```python
from build123d import *

# Parameters (mm, degrees)
ESQUISSE1_R                                        = 19
BOSS_EXTRU_1_DEPTH                                 = 2.1
ESQUISSE2_R                                        = 10
BOSS_EXTRU_2_DEPTH                                 = 6
ESQUISSE4_R                                        = 4.5
ENL_V_MAT_EXTRU_1_DEPTH                            = 21
ESQUISSE5_R                                        = 6
ENL_V_MAT_EXTRU_2_DEPTH                            = 7.2
ENL_V_MAT_EXTRU_3_DEPTH                            = 4.2
ENL_V_MAT_EXTRU_3_DEPTH_BACK                       = 10
CONG_1_R                                           = 4
ESQUISSE7_R                                        = 1.6
ENL_V_MAT_EXTRU_4_DEPTH                            = 4.2
CONG_2_R                                           = 4
ESQUISSE8_W                                        = 24.922206
ESQUISSE8_H                                        = 11.327448
ENL_V_MAT_EXTRU_5_DEPTH                            = 25
ESQUISSE9_R                                        = 4
ESQUISSE9_R_2                                      = 1.6
BOSS_EXTRU_4_DEPTH                                 = 5
CHAMBRAGE_POUR_VIS_T_TE_RONDE_BOMB_E_M_D           = 3.5
CHAMBRAGE_POUR_VIS_T_TE_RONDE_BOMB_E_M_DEPTH       = 6.948494
CHAMBRAGE_POUR_VIS_T_TE_RONDE_BOMB_E_M_CBORE_D     = 4.35
CHAMBRAGE_POUR_VIS_T_TE_RONDE_BOMB_E_M_CBORE_DEPTH = 4.8
CHAMBRAGE_POUR_VIS_T_TE_RONDE_BOMB_E_M_TIP         = 1.051506


with BuildPart() as part:
    # Esquisse1 → Boss.-Extru.1 (new body)
    with BuildSketch(Plane.XY):
        Circle(ESQUISSE1_R)
    extrude(amount=BOSS_EXTRU_1_DEPTH)

    # Esquisse2 → Boss.-Extru.2 (add)
    with BuildSketch(Plane.XY.offset(2.1)):
        Circle(ESQUISSE2_R)
    extrude(amount=BOSS_EXTRU_2_DEPTH)

    # Esquisse3 → Révolution1 (revolve)
    with BuildSketch(Plane(origin=(0, 0, 0), x_dir=(0, 0, -1), z_dir=(1, 0, 0))):
        Polygon((7.5, 0), (0, -11.25), (0, 0), align=None)
    revolve(axis=Axis((0, 0, 0), (0, 0, -1)))

    # Esquisse4 → Enlèv. mat.-Extru.1 (cut)
    with BuildSketch(Plane(origin=(0, 3.461538, -5.192308), x_dir=(0, 0.83205, 0.5547), z_dir=(0, 0.5547, -0.83205))):
        with Locations((2.600157, 0)):
            Circle(ESQUISSE4_R)
    extrude(amount=-ENL_V_MAT_EXTRU_1_DEPTH, mode=Mode.SUBTRACT)

    # Esquisse5 → Enlèv. mat.-Extru.2 (cut)
    with BuildSketch(Plane(origin=(0, 3.461538, -5.192308), x_dir=(0, 0.83205, 0.5547), z_dir=(0, 0.5547, -0.83205))):
        with Locations((2.600157, 0)):
            Circle(ESQUISSE5_R)
    extrude(amount=-ENL_V_MAT_EXTRU_2_DEPTH, mode=Mode.SUBTRACT)

    # Esquisse6 → Enlèv. mat.-Extru.3 (cut, two sides)
    with BuildSketch(Plane(origin=(0, 0, 0), x_dir=(1, 0, 0), z_dir=(0, 1, 0))) as enl_v_mat_extru_3_sk:
        with BuildLine():
            Line((2.748075, 5.66795), (0, 7.5))
            Line((0, 7.5), (-2.748075, 5.66795))
            ThreePointArc((-2.748075, 5.66795), (0, 6.5), (2.748075, 5.66795))
        make_face()
    extrude(amount=ENL_V_MAT_EXTRU_3_DEPTH, mode=Mode.SUBTRACT)
    extrude(enl_v_mat_extru_3_sk.sketch, amount=-ENL_V_MAT_EXTRU_3_DEPTH_BACK, mode=Mode.SUBTRACT)

    # Congé1
    cong_1_edges = [part.edges().sort_by_distance(p)[0] for p in [
        (-1.569953, -1.039687, -6.244664),
    ]]
    fillet(cong_1_edges, radius=CONG_1_R)

    # Esquisse7 → Enlèv. mat.-Extru.4 (cut)
    with BuildSketch(Plane(origin=(0, 0, 0), x_dir=(-1, 0, 0), z_dir=(0, 0, -1))):
        with Locations((-15, 0)):
            Circle(ESQUISSE7_R)
        with Locations((15, 0)):
            Circle(ESQUISSE7_R)
    extrude(amount=-ENL_V_MAT_EXTRU_4_DEPTH, mode=Mode.SUBTRACT)

    # Congé2
    cong_2_edges = [part.edges().sort_by_distance(p)[0] for p in [
        (0, 11.25, 0),
    ]]
    fillet(cong_2_edges, radius=CONG_2_R)

    # Esquisse8 → Enlèv. mat.-Extru.5 (cut, symmetric)
    with BuildSketch(Plane(origin=(0, 0, 0), x_dir=(1, 0, 0), z_dir=(0, 1, 0))):
        with Locations((0, 5.663724)):
            Rectangle(ESQUISSE8_W, ESQUISSE8_H)
    extrude(amount=ENL_V_MAT_EXTRU_5_DEPTH, both=True, mode=Mode.SUBTRACT)

    # Esquisse9 → Boss.-Extru.4 (add)
    with BuildSketch(Plane(origin=(0, 0, 0), x_dir=(-1, 0, 0), z_dir=(0, 0, -1))):
        with Locations((-15, 0)):
            Circle(ESQUISSE9_R)
        with Locations((-15, 0)):
            Circle(ESQUISSE9_R_2, mode=Mode.SUBTRACT)
        with Locations((15, 0)):
            Circle(ESQUISSE9_R)
        with Locations((15, 0)):
            Circle(ESQUISSE9_R_2, mode=Mode.SUBTRACT)
    extrude(amount=BOSS_EXTRU_4_DEPTH)

    # Chambrage pour vis à tête ronde bombée M21
    with Locations(Plane(origin=(15, 0, -5), x_dir=(-1, 0, 0), z_dir=(0, 0, -1))):
        with Locations((0, 0), (30, 0)):
            CounterBoreHole(CHAMBRAGE_POUR_VIS_T_TE_RONDE_BOMB_E_M_D / 2, CHAMBRAGE_POUR_VIS_T_TE_RONDE_BOMB_E_M_CBORE_D / 2, CHAMBRAGE_POUR_VIS_T_TE_RONDE_BOMB_E_M_CBORE_DEPTH, depth=CHAMBRAGE_POUR_VIS_T_TE_RONDE_BOMB_E_M_DEPTH)
            with Locations((0, 0, -(CHAMBRAGE_POUR_VIS_T_TE_RONDE_BOMB_E_M_DEPTH + CHAMBRAGE_POUR_VIS_T_TE_RONDE_BOMB_E_M_TIP / 2))):  # 118° drill point
                Cone(0, CHAMBRAGE_POUR_VIS_T_TE_RONDE_BOMB_E_M_D / 2, CHAMBRAGE_POUR_VIS_T_TE_RONDE_BOMB_E_M_TIP, mode=Mode.SUBTRACT)


solid = part.part
```
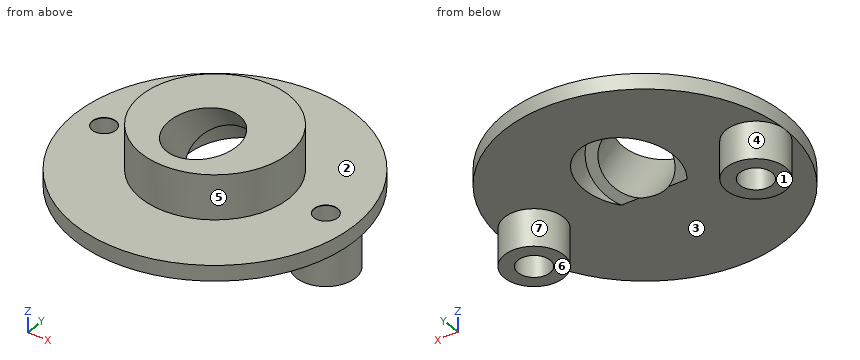
Work out the finished part from the listing and answer in its coordinate system (mm). Face numbers are marked on the shaded views. A direction names the side the tool comes from. Coordinates: 2 decimals unless noted, no trailing zeros. Loops run counter-clockwise (first coordinate to the right, second up) from the corner with the lowest first, then second, coordinate; pieces in that order, holes last. Notation, with made-up numbers: (33, -23) - (66, -23) arc R18 cw to (66, -19) - close; hole circle Ø9 at (42, 84.5). An arc over 180 degrees is marked (long way). Use a Markdown table: item, result.
Item 1: Find section D-D, the plane x = -7.5. Determine the outline of the cut face in (y, z), and give its area (3 significant figures).
Evaluation:
| item | result |
|---|---|
| outline | (-17.46, 0) - (17.46, 0) - (17.46, 2.1) - (6.61, 2.1) - (6.61, 8.1) - (-6.61, 8.1) - (-6.61, 2.1) - (-17.46, 2.1) - close |
| area | 153 mm2 |
Item 2: Find section B-B, the plane z = -2.75. Determine the outline of the cut face in (x, y) (3 decimals), and give its area (3 significant figures).
Evaluation:
| item | result |
|---|---|
| outline | circle Ø8 at (-15, 0); circle Ø8 at (15, 0); hole circle Ø4.35 at (-15, 0); hole circle Ø4.35 at (15, 0) |
| area | 70.8 mm2 |
Item 3: Find section C-C, the plane z = 1.5. State how many separate pieces and enclosed holes the cut face has, and give its area (3 significant figures).
Evaluation:
| item | result |
|---|---|
| separate pieces | 1 |
| enclosed holes | 3 |
| area | 1,000 mm2 |
Item 4: Consider probe 1 along X at (y, z) = (0, 0.4); probe 2 along Y at (x, z) = (-15, -2.7) (3 decimals); probe 3 along X at (y, z) = (0, 1.2). Determine where each line is inside the solid, lowest interval first. Write a range as from..to.
Evaluation:
| item | result |
|---|---|
| probe 1 | x = -19..-16.75, -13.25..-5.51, 5.51..13.25, 16.75..19 |
| probe 2 | y = -4..-2.175, 2.175..4 |
| probe 3 | x = -19..-16.75, -13.25..-4.06, 4.06..13.25, 16.75..19 |
Item 5: Given pin 1 Ø2 at (x, y) = (14, -0.5) entering from -Z; pin 2 Ø11.5 at (x, y) = (-8.5, 7.5) entering from -Z; pin 3 Ø2 at (x, y) = (-15, 0.5) entering from -Z; pin 4 Ø4 at (x, y) = (-13, -10) entering from +Z, each flat-ended and moving along its own axis, determine where each tip first touches the part or whether it passes through.
Evaluation:
| item | result |
|---|---|
| pin 1 | stops at z = -0.2 |
| pin 2 | stops at z = 0 |
| pin 3 | passes through |
| pin 4 | stops at z = 2.1 |
Item 6: For the marked faces 1, 2 and 3, determine the directions among +Z, -Z, +X, -X, +Y, -Y from which every point of the face is accessible in a straight line to the end or side of a thin tool.
Evaluation:
| item | result |
|---|---|
| face 1 | -Z, +X, -X, +Y, -Y |
| face 2 | +Z |
| face 3 | -Z |
Item 7: The mould has two halves that part along X. Classify the marked faces 4, 5, 6 and 7: +X half, -X half, draft (parallel to the pull), parting line (faces both ways), or undercut.
Evaluation:
| item | result |
|---|---|
| face 4 | undercut |
| face 5 | parting line |
| face 6 | draft |
| face 7 | undercut |
